```python
from build123d import *

# Parameters (mm, degrees)
PAD_DEPTH     = 1.3
SKETCH001_R   = 2.011692
SKETCH001_W   = 32
SKETCH001_H   = 29
SKETCH001_W_2 = 7
SKETCH001_H_2 = 5
SKETCH001_W_3 = 14
SKETCH001_H_3 = 15.5
PAD001_DEPTH  = 1.75
SKETCH002_W   = 12
SKETCH002_H   = 8
SKETCH002_W_2 = 14.5
SKETCH002_H_2 = 6
PAD002_DEPTH  = 5
SKETCH003_W   = 4.4
SKETCH003_H   = 4.4
SKETCH003_W_2 = 4.3
SKETCH003_H_2 = 3.2
SKETCH003_W_3 = 7.5
SKETCH003_H_3 = 5.75
PAD003_DEPTH  = 3
SKETCH004_W   = 4.2
SKETCH004_H   = 3.2
PAD004_DEPTH  = 3
SKETCH005_R   = 1.6
POCKET_DEPTH  = 6.301


with BuildPart() as part:
    # Sketch → Pad (new body)
    with BuildSketch(Plane.XZ):
        with BuildLine():
            Line((-53.25, 48.1), (-1.75, 48.1))
            ThreePointArc((0, 46.35), (-0.512563, 47.587437), (-1.75, 48.1))
            Line((0, 46.35), (0, 1.75))
            ThreePointArc((-1.75, 0), (-0.512563, 0.512563), (0, 1.75))
            Line((-1.75, 0), (-53.25, 0))
            ThreePointArc((-55, 1.75), (-54.487437, 0.512563), (-53.25, 0))
            Line((-55, 1.75), (-55, 46.35))
            ThreePointArc((-53.25, 48.1), (-54.487437, 47.587437), (-55, 46.35))
        make_face()
    extrude(amount=PAD_DEPTH)

    # Sketch001 (on Face9 of Pad) → Pad001 (join)
    with BuildSketch(Plane(origin=(0, 0, 0), x_dir=(1, 0, 0), z_dir=(0, 1, 0))):
        with Locations((-52, -24.1)):
            Circle(SKETCH001_R)
        with Locations((-52, -11.6)):
            Circle(SKETCH001_R)
        with Locations((-52, -36.6)):
            Circle(SKETCH001_R)
        with Locations((-32.5, -24.1)):
            Rectangle(SKETCH001_W, SKETCH001_H)
        with Locations((-29.49, -43.86)):
            Rectangle(SKETCH001_W_2, SKETCH001_H_2)
        with Locations((-7.5, -37.35)):
            Rectangle(SKETCH001_W_3, SKETCH001_H_3)
    extrude(amount=PAD001_DEPTH)

    # Sketch002 (on Face5 of Pad001) → Pad002 (join)
    with BuildSketch(Plane.XZ.offset(1.3)):
        with Locations((-41, 43.1)):
            Rectangle(SKETCH002_W, SKETCH002_H)
        with Locations((-27.25, 43.1)):
            Rectangle(SKETCH002_W, SKETCH002_H)
        with Locations((-13.5, 43.1)):
            Rectangle(SKETCH002_W, SKETCH002_H)
        with Locations((-41, 5)):
            Rectangle(SKETCH002_W, SKETCH002_H)
        with Locations((-27.25, 5)):
            Rectangle(SKETCH002_W, SKETCH002_H)
        with Locations((-13.5, 5)):
            Rectangle(SKETCH002_W, SKETCH002_H)
        with Locations((-6, 30.995757)):
            Rectangle(SKETCH002_W_2, SKETCH002_H_2)
    extrude(amount=PAD002_DEPTH)

    # Sketch003 (on Face5 of Pad002) → Pad003 (join)
    with BuildSketch(Plane.XZ.offset(1.3)):
        with Locations((-2.437883, 42.9)):
            Rectangle(SKETCH003_W, SKETCH003_H)
        with Locations((-3.15, 37.5)):
            Rectangle(SKETCH003_W_2, SKETCH003_H_2)
        with Locations((-2.75, 16.375)):
            Rectangle(SKETCH003_W_3, SKETCH003_H_3)
        with Locations((-3.15, 9.6)):
            Rectangle(SKETCH003_W_2, SKETCH003_H_2)
    extrude(amount=PAD003_DEPTH)

    # Sketch004 (on Face4 of Pad003) → Pad004 (join)
    with BuildSketch(Plane(origin=(0, 0, 0), x_dir=(1, 0, 0), z_dir=(0, 1, 0))):
        with Locations((-9.85, -3.35)):
            Rectangle(SKETCH004_W, SKETCH004_H)
    extrude(amount=PAD004_DEPTH)

    # Sketch005 (on Face4 of Pad004) → Pocket (cut, through all)
    with BuildSketch(Plane(origin=(0, 0, 0), x_dir=(1, 0, 0), z_dir=(0, 1, 0))):
        with Locations((-3.2, -3.2)):
            Circle(SKETCH005_R)
        with Locations((-51.8, -44.9)):
            Circle(SKETCH005_R)
    extrude(amount=-POCKET_DEPTH, mode=Mode.SUBTRACT)


solid = part.part
```
Here's how the part is built. I have some questions about the finished solid (model axes, mm). A direction names the side the tool comes from. Coordinates: 2 decimals unless noted, no trailing zeros. Loops run counter-clockwise (first coordinate to the right, second up) from the corner with the lowest first, then second, coordinate; pieces in that order, holes last. Notation, with made-up numbers: M 77.25,-40 L 87.25,-40 A29 ccw 87.25,-11 Z; hole C 5,12.25 d2. An arc over 180 degrees is marked long. One line per item, written item: value.
1. Please list where these lines run through material, in increasing order: probe 1 along Z at (x, y) = (-12, -2.5); probe 2 along X at (y, z) = (-0.3, 3.2); probe 3 along X at (y, z) = (-0.65, 44.9).
Geometry says:
probe 1: z = 1 to 9, 28 to 34, 39.1 to 47.1
probe 2: x = -55 to -4.8, -1.6 to 0
probe 3: x = -55 to -53.4, -50.2 to 0
2. Will these pins go through, and if not, where does the flat tip stop? pin 1 Ø1 at (y, z) = (-2, 33) entering from -X; pin 2 Ø1.5 at (y, z) = (-4, 42) entering from +X; pin 3 Ø1 at (y, z) = (1, 31) entering from -X.
Geometry says:
pin 1: stops at x = -13.25
pin 2: stops at x = -0.24
pin 3: stops at x = -48.5
3. Imagine slicing it at C-C (x = -44.5). List the corners of the cut face in (y, z) for me, and give its area (3 significant figures).
Geometry says:
outline: M -6.3,1 L -1.3,1 L -1.3,0 L 0,0 L 0,9.6 L 1.75,9.6 L 1.75,38.6 L 0,38.6 L 0,48.1 L -1.3,48.1 L -1.3,47.1 L -6.3,47.1 L -6.3,39.1 L -1.3,39.1 L -1.3,9 L -6.3,9 Z
area: 193 mm2
4. Imagine slicing it at D-D (x = -51.8). List the corners of the cut face in (y, z) for me.
Geometry says:
outline: M -1.3,0 L 0,0 L 0,9.6 L 1.75,9.6 L 1.75,13.6 L 0,13.6 L 0,22.1 L 1.75,22.1 L 1.75,26.1 L 0,26.1 L 0,34.6 L 1.75,34.6 L 1.75,38.6 L 0,38.6 L 0,43.3 L -1.3,43.3 Z; M -1.3,46.5 L 0,46.5 L 0,48.1 L -1.3,48.1 Z
5. Imagine slicing it at B-B (z = 36.6). List the corners of the cut face in (x, y) for me.
Geometry says:
outline: M -55,-1.3 L -5.3,-1.3 L -5.3,-4.3 L -1,-4.3 L -1,-1.3 L 0,-1.3 L 0,0 L -0.5,0 L -0.5,1.75 L -14.5,1.75 L -14.5,0 L -16.5,0 L -16.5,1.75 L -48.5,1.75 L -48.5,0 L -49.99,0 L -49.99,1.75 L -54.01,1.75 L -54.01,0 L -55,0 Z
6. Thinking about a two-plate mould opening in Z: for faces 6 (the flat face through (-47, -4, 43)), 7 (the flat face through (-28, -1, 48.1)), 8 (the flat face through (-14, -4, 39.1)), which applies, +Z half, -Z half, draft (parallel to the pull), parting line (faces both ways), or undercut?
Geometry says:
face 6: draft
face 7: +Z half
face 8: undercut
7. On a 3-axis mill with a long thin cutter (end or side, diameter ignored), from which of +Z, -Z, +X, -X, +Y, -Y can I reach the whole of each face in a straight line? I mean faces 1 (the flat face through (-3, -3, 8)), 2 (the flat face through (-6.5, -3, 16)), 3 (the flat face through (-6, -4, 27.996)), 4 (the flat face through (-19.5, -4, 5)), 5 (the flat face through (-1, -3, 37)). Say none if no direction works.
Geometry says:
face 1: -Z, +X, -Y
face 2: -Z, -X, -Y
face 3: +X, -X, -Y
face 4: +Z, -Z, -Y
face 5: +X, -Y
8. Imagine slicing it at A-A (y = -5.5). List the corners of the cut face in (x, z) for me, and give its area (3 significant figures).
Geometry says:
outline: M -47,1 L -35,1 L -35,9 L -47,9 Z; M -47,39.1 L -35,39.1 L -35,47.1 L -47,47.1 Z; M -33.25,1 L -21.25,1 L -21.25,9 L -33.25,9 Z; M -33.25,39.1 L -21.25,39.1 L -21.25,47.1 L -33.25,47.1 Z; M -19.5,1 L -7.5,1 L -7.5,9 L -19.5,9 Z; M -19.5,39.1 L -7.5,39.1 L -7.5,47.1 L -19.5,47.1 Z; M -13.25,28 L 1.25,28 L 1.25,34 L -13.25,34 Z
area: 663 mm2
